from build123d import *

# Parameters (mm, degrees)
F0_W     = 32
F0_H     = 46
F0_W_2   = 8
F0_H_2   = 40
F0_R     = 2
F1_DEPTH = 4
F2_W     = 4
F2_H     = 4
F2_H_2   = 2
F3_DEPTH = 8
F4_W     = 4
F4_H     = 22
F5_DEPTH = 4


with BuildPart() as f1:
    # F0 (on Front) → F1 (new body)
    with BuildSketch(Plane.XZ):
        with Locations((0, -23)):
            Rectangle(F0_W, F0_H)
        with Locations((-8, -24)):
            Rectangle(F0_W_2, F0_H_2, mode=Mode.SUBTRACT)
        with Locations((0, -40)):
            Circle(F0_R, mode=Mode.SUBTRACT)
        with Locations((0, -27)):
            Circle(F0_R, mode=Mode.SUBTRACT)
        with Locations((8, -24)):
            Rectangle(F0_W_2, F0_H_2, mode=Mode.SUBTRACT)
    extrude(amount=F1_DEPTH)

    # F2 (on face) → F3 (join)
    with BuildSketch(Plane.XZ.offset(4)):
        with Locations((-14, -2)):
            Rectangle(F2_W, F2_H)
        with Locations((14, -2)):
            Rectangle(F2_W, F2_H)
        with Locations((0, -2)):
            Rectangle(F2_W, F2_H)
        with Locations((-14, -26)):
            Rectangle(F2_W, F2_H)
        with Locations((14, -26)):
            Rectangle(F2_W, F2_H)
        with Locations((-14, -45)):
            Rectangle(F2_W, F2_H_2)
        with Locations((14, -45)):
            Rectangle(F2_W, F2_H_2)
    extrude(amount=F3_DEPTH)

    # F4 (on face) → F5 (join)
    with BuildSketch(Plane.XZ.offset(12)):
        with Locations((-14, -35)):
            Rectangle(F4_W, F4_H)
        with Locations((14, -35)):
            Rectangle(F4_W, F4_H)
    extrude(amount=-F5_DEPTH)


solid = f1.part
Model file for the job. Use its own axes, mm. A direction names the side the tool comes from. Give positions to 0.01 mm unless a question says otherwise; leave off trailing zeros. Loops run counter-clockwise (first coordinate to the right, second up) from the corner with the lowest first, then second, coordinate; pieces in that order, holes last. Notation, with made-up numbers: (-6.5, -34) -> (31.5, -34) arc R33 cw to (31.5, 2) -> close; hole circle Ø2 at (27.5, 71.5). An arc over 180 degrees is marked (long way). Use a Markdown table: item, result. Add a question column.
(1) Drop flat-ended pins along their axis: pin 1 Ø1.2 at (x, z) = (-15, -16.5) entering from -Y; pin 2 Ø3 at (x, y) = (0, -9.5) entering from -Z. Give the stop position or say it passes through.
(2) Slice it at C-C on z = -40. List the corners of the cut face in (x, y).
(3) Mould opens along X. For faces 4 (the flat face through (-14, -8, -36)), 5 (the flat face through (12, -3, -30)), 6 (the flat face through (16, -3, -23)) say: +X half, -X half, draft (parallel to the pull), parting line (faces both ways), or undercut.
(4) Slice it at B-B on x = 10. List the corners of the cut face in (y, z), and give its area (3 significant figures).
(5) Wall check: line 1 along X through (y, z) = (-3.25, -34); line 2 along Z through (x, y) = (0, -2.4); line 3 along Z through (x, y) = (14, -10.25). Give the ranges that are in metal, low to high.
(6) Slice it at A-A on y = -9.75. List the corners of the cut face in (x, z), and give its area (3 significant figures).
(7) Tool access for faces 1 (the flat face through (-8, -2, -44)), 2 (the flat face through (-14, -8, -4)), 3 (the flat face through (-2, -8, -2)): list every direction of +Z, -Z, +X, -X, +Y, -Y with a clear straight run to the whole face (end or side of a thin tool).
(8) Slice it at D-D on y = -2. List the corners of the cut face in (x, z).
Filled sheet:
| question | item | result |
|---|---|---|
| 1 | pin 1 | y = -4 |
| 1 | pin 2 | z = -4 |
| 2 | outline | (-16, -12) -> (-12, -12) -> (-12, -8) -> (-16, -8) -> close; (-16, -4) -> (-12, -4) -> (-12, 0) -> (-16, 0) -> close; (-4, -4) -> (-2, -4) -> (-2, 0) -> (-4, 0) -> close; (2, -4) -> (4, -4) -> (4, 0) -> (2, 0) -> close; (12, -12) -> (16, -12) -> (16, -8) -> (12, -8) -> close; (12, -4) -> (16, -4) -> (16, 0) -> (12, 0) -> close |
| 3 | face 4 | draft |
| 3 | face 5 | undercut |
| 3 | face 6 | +X half |
| 4 | outline | (-4, -46) -> (0, -46) -> (0, -44) -> (-4, -44) -> close; (-4, -4) -> (0, -4) -> (0, 0) -> (-4, 0) -> close |
| 4 | area | 24.0 mm2 |
| 5 | line 1 | -16 to -12, -4 to 4, 12 to 16 |
| 5 | line 2 | -46 to -42, -38 to -29, -25 to 0 |
| 5 | line 3 | -46 to -24, -4 to 0 |
| 6 | outline | (-16, -46) -> (-12, -46) -> (-12, -24) -> (-16, -24) -> close; (-16, -4) -> (-12, -4) -> (-12, 0) -> (-16, 0) -> close; (-2, -4) -> (2, -4) -> (2, 0) -> (-2, 0) -> close; (12, -46) -> (16, -46) -> (16, -24) -> (12, -24) -> close; (12, -4) -> (16, -4) -> (16, 0) -> (12, 0) -> close |
| 6 | area | 224 mm2 |
| 7 | face 1 | +Y, -Y |
| 7 | face 2 | +X, -X, -Y |
| 7 | face 3 | +Z, -Z, -Y |
| 8 | outline | (-16, -46) -> (16, -46) -> (16, 0) -> (-16, 0) -> close; hole (-12, -44) -> (-4, -44) -> (-4, -4) -> (-12, -4) -> close; hole circle Ø4 at (0, -40); hole circle Ø4 at (0, -27); hole (4, -44) -> (12, -44) -> (12, -4) -> (4, -4) -> close |
